Could you check a few things on this model? Use its own coordinates, in mm. A direction names the side the tool comes from. Round coordinates to 2 decimals unless told otherwise and drop trailing zeros. Loops run counter-clockwise (first coordinate to the right, second up) from the corner with the lowest first, then second, coordinate; pieces in that order, holes last. Notation, with made-up numbers: (21.5, -19) -> (40.5, -19) arc R33 ccw to (40.5, 14) -> close; hole circle Ø5 at (17, 22.5). An arc over 180 degrees is marked (long way). Write each question's results on one line, items separated by ' | '. Start each with the question number.
1) Imagine slicing it at B-B, the plane z = -4. List the corners of the cut face in (x, y) for me.
2) We'd pull the mould along Y, two halves only. Please class faces 3 (the flat face through (-22.95, 22.78, 12.9)), 4 (the flat face through (0, 15, 0)), 5 (the flat face through (-1, 0, -1)): pulls with the +Y half, pulls with the -Y half, needs draft (parallel to the pull), parting line crosses it, or undercut.
3) Which directions (+Z, -Z, +X, -X, +Y, -Y) give clear straight access to the entire face, cutting with the end or side of a thin tool? Please do faces 1 (the flat face through (22.65, 22.78, 13.42)), 2 (the flat face through (0, 45, 0)).
4) Imagine slicing it at D-D, the plane x = -14. List the corners of the cut face in (y, z) for me, plus the area to 3 significant figures.
5) For P1, Ø2, axis at x = -0.5, y = 63.5, coming from the -Z side; P2, Ø1.5, axis at y = 56, z = -7, coming from the +X side; P3, Ø8, axis at x = -23, z = 7, coming from the -Y side; P4, Ø15, axis at x = -1.5, y = 36, coming from the +Z side, each with a flat end and sliding along its axis, tell me the tip position at first contact or that it passes through.
6) Imagine slicing it at C-C, the plane x = -5. List the corners of the cut face in (y, z) for me.
7) If I drill on probe 1 along Y at (x, z) = (-19, -5.5); probe 2 along Z at (x, y) = (-2.5, 27); probe 3 along Y at (x, z) = (-12.5, -1.5), over which ranges is the centre line in solid material (lowest first)?
8) Imagine slicing it at A-A, the plane y = 25. List the corners of the cut face in (x, z) for me.
Autodesk Inventor part; units mm, degrees
ref_plane "YZ Plane" through (0, 0, 0) normal (1, 0, 0) x (0, 1, 0)
ref_plane "XZ Plane" through (0, 0, 0) normal (0, 1, 0) x (-1, 0, 0)
ref_plane "XY Plane" through (0, 0, 0) normal (0, 0, 1) x (1, 0, 0)
sketch "Эскиз1" plane through (0, 0, 0) normal (0, 1, 0) x (-1, 0, 0)
  line L0 (42.5, 0) -> (21.25, -36.8061)
  line L1 (21.25, -36.8061) -> (-21.25, -36.8061)
  line L2 (-21.25, -36.8061) -> (-42.5, 0)
  line L3 (-42.5, 0) -> (-21.25, 36.8061)
  line L4 (-21.25, 36.8061) -> (21.25, 36.8061)
  line L5 (21.25, 36.8061) -> (42.5, 0)
  point P0 (0, 0)
  point P1 (0, 0)
  dimension "d0" = 85
sketch "Эскиз2" plane through (0, 0, 0) normal (1, 0, 0) x (0, 1, 0)
  point P0 (0, 0)
  point P1 (80, 0)
  dimension "d1" = 80
loft "Лофт1" add profiles "Эскиз1" section 2 point at (0, 80, 0)
sketch "Эскиз3" plane through (0, 0, 0) normal (1, 0, 0) x (0, 1, 0)
  line L0 (15, -12.5) -> (45, -12.5)
  line L1 (45, -12.5) -> (45, 12.5)
  line L2 (45, 12.5) -> (15, 12.5)
  line L3 (15, 12.5) -> (15, -12.5)
  line L4 (0, 0) -> (80, 0)
  line L5 (15, -12.5) -> (45, 12.5) construction
  line L6 (45, -12.5) -> (15, 12.5) construction
  line L7 (0, 0) -> (0, 36.8061)
  point P0 (30, 0)
  dimension "d6" = 30
  dimension "d7" = 25
  dimension "d8" = 15
extrude "Выдавливание1" cut sketch "Эскиз3" along normal through all both and the other way through all
properties part number "Пирамида"
Checked values:
1) outline: (-40.19, 0) -> (40.19, 0) -> (32.22, 15) -> (-32.22, 15) -> close; (-16.28, 45) -> (16.28, 45) -> (2.31, 71.31) -> (-2.31, 71.31) -> close
2) face 3: pulls with the +Y half | face 4: undercut | face 5: pulls with the -Y half
3) face 1: +Z, +X, +Y | face 2: +X, -X
4) outline: (0, -36.81) -> (27.29, -24.25) -> (40.06, -12.5) -> (15, -12.5) -> (15, 12.5) -> (40.06, 12.5) -> (27.29, 24.25) -> (0, 36.81) -> close; (45, -7.96) -> (53.65, 0) -> (45, 7.96) -> close | area: 1,580 mm^2
5) P1: z = -8.05 | P2: x = 9.3 | P3: y = 0 | P4: z = 23.69
6) outline: (0, -36.81) -> (61.18, -8.66) -> (70.59, 0) -> (61.18, 8.66) -> (0, 36.81) -> close; hole (15, -12.5) -> (45, -12.5) -> (45, 12.5) -> (15, 12.5) -> close
7) probe 1: 0 to 15 | probe 2: -24.38 to -12.5, 12.5 to 24.38 | probe 3: 0 to 15, 45 to 54.84
8) outline: (-22, -12.5) -> (-14.61, -25.3) -> (14.61, -25.3) -> (22, -12.5) -> close; (-22, 12.5) -> (22, 12.5) -> (14.61, 25.3) -> (-14.61, 25.3) -> close
